from build123d import *

# Parameters (mm, degrees)
BOSS_EXTRUDE1_DEPTH = 16.5
BOSS_EXTRUDE7_DEPTH = 1
BOSS_EXTRUDE8_DEPTH = 1
SKETCH9_R           = 1.75
BOSS_EXTRUDE9_DEPTH = 7.909853
CUT_EXTRUDE2_START  = -3.590147425
SKETCH11_R          = 3.25
CUT_EXTRUDE2_DEPTH  = 3.590147425
CUT_EXTRUDE3_START  = -18.5
SKETCH12_W          = 5.25
SKETCH12_H          = 1
SKETCH12_W_2        = 1.5
CUT_EXTRUDE3_DEPTH  = 18.5
FILLET1_R           = 3


with BuildPart() as part:
    # Sketch1 → Boss-Extrude1 (new body)
    with BuildSketch(Plane(origin=(0, 0, 0), x_dir=(1, 0, 0), z_dir=(0, 1, 0))):
        Polygon((-7.219839172, 4.25), (-5, 4.25), (8, 4.25), (8, -4.25), (-5, -4.25), (-7.219839172, -4.25), (-5.583475536, -5.75), (9.5, -5.75), (9.5, 5.75), (-5.583475536, 5.75), align=None)
        Polygon((-8, -4.25), (-8, -3.534852575), (-9.5, -2.159852575), (-9.5, -5.75), (-5.583475536, -5.75), (-7.219839172, -4.25), align=None)
        Polygon((-8, -1.5), (-8, 1.5), (-8, 3.534852575), (-9.5, 2.159852575), (-9.5, -2.159852575), (-8, -3.534852575), align=None)
        Polygon((-8, 1.5), (-5, 4.25), (-7.219839172, 4.25), (-8, 3.534852575), align=None)
        Polygon((-5, -4.25), (-8, -1.5), (-8, -3.534852575), (-7.219839172, -4.25), align=None)
        Polygon((-7.219839172, -4.25), (-8, -3.534852575), (-8, -4.25), align=None)
    extrude(amount=BOSS_EXTRUDE1_DEPTH)

    # Sketch7 → Boss-Extrude7 (add)
    # profile 1 of 2: a face of its own
    with BuildSketch(Plane(origin=(0, 16.5, 0), x_dir=(1, 0, 0), z_dir=(0, 1, 0))):
        Polygon((9.5, 5.75), (-5.583475536, 5.75), (-9.5, 2.159852575), (-9.5, -5.75), (9.5, -5.75), align=None)
        Polygon((8, -4.25), (-5, -4.25), (-8, -1.5), (-8, 1.5), (-5, 4.25), (8, 4.25), align=None, mode=Mode.SUBTRACT)
    # profile 2 of 2: a face of its own
    with BuildSketch(Plane(origin=(0, 16.5, 0), x_dir=(1, 0, 0), z_dir=(0, 1, 0))):
        Polygon((-4.922203262, 4.05), (7.8, 4.05), (8, 4.05), (8, 4.25), (-5, 4.25), (-8, 1.5), (-8, -1.5), (-5, -4.25), (8, -4.25), (8, -4.05), (7.8, -4.05), (-4.922203262, -4.05), (-7.8, -1.412019657), (-7.8, 1.412019657), align=None)
    extrude(amount=BOSS_EXTRUDE7_DEPTH)

    # Sketch8 → Boss-Extrude8 (add)
    with BuildSketch(Plane.XZ):
        Polygon((-9.5, -2.159852575), (-5.583475536, -5.75), (9.5, -5.75), (9.5, 5.75), (-9.5, 5.75), align=None)
        Polygon((8, 4.05), (-4.922203262, 4.05), (-7.8, 1.412019657), (-7.8, -1.412019657), (-4.922203262, -4.05), (8, -4.05), align=None, mode=Mode.SUBTRACT)
    extrude(amount=BOSS_EXTRUDE8_DEPTH)

    # Sketch9 → Boss-Extrude9 (add)
    # profile 1 of 4: a face of its own
    with BuildSketch(Plane.XY.offset(5.75)):
        with BuildLine():
            Line((-9.5, 0.438262309), (-9.5, 5.561737691))
            ThreePointArc((-9.5, 5.561737691), (-12.925219281, 5.920830361), (-14.75, 3))
            ThreePointArc((-14.75, 3), (-12.925219281, 0.079169639), (-9.5, 0.438262309))
        make_face()
        with Locations((-11.5, 3)):
            Circle(SKETCH9_R, mode=Mode.SUBTRACT)
    # profile 2 of 4: a face of its own
    with BuildSketch(Plane.XY.offset(5.75)):
        with BuildLine():
            ThreePointArc((14.75, 3), (12.925219281, 5.920830361), (9.5, 5.561737691))
            Line((9.5, 5.561737691), (9.5, 0.438262309))
            ThreePointArc((9.5, 0.438262309), (12.925219281, 0.079169639), (14.75, 3))
        make_face()
        with Locations((11.5, 3)):
            Circle(SKETCH9_R, mode=Mode.SUBTRACT)
    # profile 3 of 4: a face of its own
    with BuildSketch(Plane.XY.offset(5.75)):
        with BuildLine():
            Line((-9.5, -1), (-9.5, 0.438262309))
            ThreePointArc((-9.5, 0.438262309), (-12.925219281, 0.079169639), (-14.75, 3))
            Line((-14.75, 3), (-14.75, -1))
            Line((-14.75, -1), (-9.5, -1))
        make_face()
    # profile 4 of 4: a face of its own
    with BuildSketch(Plane.XY.offset(5.75)):
        with BuildLine():
            ThreePointArc((14.75, 3), (12.925219281, 0.079169639), (9.5, 0.438262309))
            Line((9.5, 0.438262309), (9.5, -1))
            Line((9.5, -1), (14.75, -1))
            Line((14.75, -1), (14.75, 3))
        make_face()
    extrude(amount=-BOSS_EXTRUDE9_DEPTH)

    # Sketch11 → Cut-Extrude2 (cut)
    with BuildSketch(Plane(origin=(0, 0, -5.75), x_dir=(-1, 0, 0), z_dir=(0, 0, -1)).offset(CUT_EXTRUDE2_START)):
        with Locations((-11.5, 3)):
            Circle(SKETCH11_R)
        with Locations((11.5, 3)):
            Circle(SKETCH11_R)
    extrude(amount=CUT_EXTRUDE2_DEPTH, mode=Mode.SUBTRACT)

    # Sketch12 → Cut-Extrude3 (cut)
    with BuildSketch(Plane(origin=(0, 17.5, 0), x_dir=(1, 0, 0), z_dir=(0, 1, 0)).offset(CUT_EXTRUDE3_START)):
        with Locations((12.125, -3.55)):
            Rectangle(SKETCH12_W, SKETCH12_H)
        with Locations((8.75, -3.55)):
            Rectangle(SKETCH12_W_2, SKETCH12_H)
    extrude(amount=CUT_EXTRUDE3_DEPTH, mode=Mode.SUBTRACT)

    # Fillet1
    # the kernel refuses this fillet: 3 mm, written as the material it adds along each edge
    with BuildSketch(Plane(origin=(-9.5, 5.561737691, 5.75), x_dir=(0, 1, 0), z_dir=(0, 0, -1))) as fillet1_piece_1_section:
        with BuildLine():
            CenterArc((3.607743648, -3), FILLET1_R, 90, 80.793103779)
            ThreePointArc((0.646392605, -2.52), (0.5863481, -1.192500248), (0, 0))
            Line((0, 0), (3.607743648, 0))
        make_face()
    fillet1_piece_1 = extrude(amount=16.929211695, mode=Mode.PRIVATE)
    fillet1_piece_1 = split(fillet1_piece_1, bisect_by=Plane(origin=(-10.050248637, 6.751557593, -2.159853), z_dir=(0, 0, 1)), keep=Keep.TOP, mode=Mode.PRIVATE)
    add(fillet1_piece_1)
    with BuildSketch(Plane(origin=(9.5, 5.561737691, 12.06935912), x_dir=(0.968641781969148, 0.24846146225045335, 0), z_dir=(0, 0, -1))) as fillet1_piece_2_section:
        with BuildLine():
            CenterArc((3.802310608, -2.749226849), FILLET1_R, 113.593384333, 80.793103779)
            Line((0.896385262, -3.494611236), (0, 0))
            ThreePointArc((0, 0), (1.300790471, -0.271670913), (2.601580942, 0))
        make_face()
    fillet1_piece_2 = extrude(amount=23.248570816, mode=Mode.PRIVATE)
    fillet1_piece_2 = split(fillet1_piece_2, bisect_by=Plane(origin=(10.078407886, 6.738604844, 5.75), z_dir=(0, 0, -1)), keep=Keep.TOP, mode=Mode.PRIVATE)
    fillet1_piece_2 = split(fillet1_piece_2, bisect_by=Plane(origin=(10.078407886, 6.738604844, 4.05), z_dir=(0, 0, 1)), keep=Keep.TOP, mode=Mode.PRIVATE)
    add(fillet1_piece_2)
    with BuildSketch(Plane(origin=(9.5, 5.561737691, 3.05), x_dir=(0.9686417819691505, 0.24846146225044377, 0), z_dir=(0, 0, -1))) as fillet1_piece_3:
        with BuildLine():
            CenterArc((3.802310608, -2.749226849), FILLET1_R, 113.593384333, 80.793103779)
            Line((0.896385262, -3.494611236), (0, 0))
            ThreePointArc((0, 0), (1.300790471, -0.271670913), (2.601580942, 0))
        make_face()
    extrude(amount=5.209852575)
    with BuildSketch(Plane(origin=(9.5, 5.561737691, 5.75), x_dir=(0.9686417819691505, 0.24846146225044377, 0), z_dir=(0, 0, -1))) as fillet1_piece_4:
        with BuildLine():
            CenterArc((3.802310608, -2.749226849), FILLET1_R, 113.593384333, 80.793103779)
            Line((0.896385262, -3.494611236), (0, 0))
            ThreePointArc((0, 0), (1.300790471, -0.271670913), (2.601580942, 0))
        make_face()
    extrude(amount=1.7)
    with BuildSketch(Plane(origin=(9.5, 5.561737691, 14.76935912), x_dir=(0.968641781969148, 0.24846146225045335, 0), z_dir=(0, 0, -1))) as fillet1_piece_5_section:
        with BuildLine():
            CenterArc((3.802310608, -2.749226849), FILLET1_R, 113.593384333, 80.793103779)
            Line((0.896385262, -3.494611236), (0, 0))
            ThreePointArc((0, 0), (1.300790471, -0.271670913), (2.601580942, 0))
        make_face()
    fillet1_piece_5 = extrude(amount=19.738718241, mode=Mode.PRIVATE)
    fillet1_piece_5 = split(fillet1_piece_5, bisect_by=Plane(origin=(10.078407886, 6.738604844, 3.05), z_dir=(0, 0, -1)), keep=Keep.TOP, mode=Mode.PRIVATE)
    fillet1_piece_5 = split(fillet1_piece_5, bisect_by=Plane(origin=(10.078407886, 6.738604844, -2.159852575), z_dir=(0, 0, 1)), keep=Keep.TOP, mode=Mode.PRIVATE)
    add(fillet1_piece_5)


solid = part.part
Read the model definition and answer for the solid it produces. Units are mm, in the model's axes. A direction names the side the tool comes from. Round coordinates to 2 decimals unless told otherwise and drop trailing zeros. Write each loop counter-clockwise with the first axis right and the second up, starting at its lowest first coordinate (ties: lowest second). Pieces come first, ordered by that corner, then holes.
1. Given pin 1 Ø6 at (y, z) = (7.5, 0.5) entering from -X; pin 2 Ø1.5 at (y, z) = (9, 0.5) entering from +X; pin 3 Ø4 at (x, z) = (1.5, -0.5) entering from +Y; pin 4 Ø2 at (y, z) = (8, -3) entering from +X, each flat-ended and moving along its own axis, determine where each tip first touches the part or whether it passes through.
2. The part is cut by section D-D, the plane x = 12.75. Determine the outline of the cut face in (y, z), then the cut area to 3 significant figures.
3. Which of the six approach directions +Z, -Z, +X, -X, +Y, -Y give full straight-line access (tool end or side, diameter ignored) to faces 4 (the face through (-8, 8, 0)), 5 (the face through (10, 6, 3.05)), 6 (the face through (-8.25, 3.04, -2.67))?
4. Determine the mould class of faces 1 (the face through (-6.381, -0.493, -2.713)), 2 (the face through (13.996, 5.082, 0.482)), 3 (the face through (12.31, 1.45, 0.48)) for opening direction Y: pulls with the +Y half, pulls with the -Y half, needs draft (parallel to the pull), parting line crosses it, or undercut.
5. The part is cut by section B-B, the plane x = -6. Determine the outline of the cut face in (y, z).
6. The part is cut by section A-A, the plane z = 0. Determine the outline of the cut face in (x, y), then the cut area to 3 significant figures.
7. The part is cut by section C-C, the plane y = 14.25. Determine the outline of the cut face in (x, z).
8. Straight lines are drawn through the part: L1, parallel to Z at x = 7.25, y = 16.75; L2, parallel to Z at x = 2, y = 10; L3, parallel to Y at x = 11.5, z = -1.05. For each, find the intervals that lie inside material, in ascending order.
Values:
1. pin 1: stops at x = -14.38
1. pin 2: stops at x = 9.64
1. pin 3: passes through
1. pin 4: stops at x = 10.04
2. outline: (-1, -2.16) - (1.78, -2.16) - (1.78, 3.05) - (-1, 3.05) - close; (-1, 4.05) - (1.78, 4.05) - (1.78, 5.75) - (-1, 5.75) - close; (4.22, -2.16) - (6, -2.16) - (6, 3.05) - (4.22, 3.05) - close; (4.22, 4.05) - (6, 4.05) - (6, 5.75) - (4.22, 5.75) - close
2. area: 31.4 mm2
3. face 4: none
3. face 5: +X, +Y, -Y
3. face 6: -Z, -X
4. face 1: needs draft
4. face 2: pulls with the +Y half
4. face 3: undercut
5. outline: (-1, -5.37) - (17.5, -5.37) - (17.5, -3.06) - (16.5, -3.06) - (16.5, -3.33) - (0, -3.33) - (0, -3.06) - (-1, -3.06) - close; (-1, 3.06) - (0, 3.06) - (0, 3.33) - (16.5, 3.33) - (16.5, 3.06) - (17.5, 3.06) - (17.5, 5.75) - (-1, 5.75) - close
6. outline: (-14.75, -1) - (-7.8, -1) - (-7.8, 0) - (-8, 0) - (-8, 16.5) - (-7.8, 16.5) - (-7.8, 17.5) - (-9.5, 17.5) - (-9.5, 9.17) arc R3 cw to (-12.02, 6.21) arc R3.25 ccw to (-14.75, 3) - close; (8, -1) - (14.75, -1) - (14.75, 3) arc R3.25 ccw to (12.02, 6.21) arc R3 cw to (9.5, 9.17) - (9.5, 17.5) - (8, 17.5) - close; hole circle Ø3.5 at (-11.5, 3); hole circle Ø3.5 at (11.5, 3)
6. area: 112 mm2
7. outline: (-9.5, -2.16) - (-5.58, -5.75) - (9.5, -5.75) - (9.5, 3.05) - (8, 3.05) - (8, -4.25) - (-5, -4.25) - (-8, -1.5) - (-8, 1.5) - (-5, 4.25) - (8, 4.25) - (8, 4.05) - (9.5, 4.05) - (9.5, 5.75) - (-9.5, 5.75) - close
8. L1: z = -5.75 to -4.05, 4.05 to 5.75
8. L2: z = -5.75 to -4.25, 4.25 to 5.75
8. L3: y = -1 to 1.25, 4.75 to 6.34
